Autodesk Inventor part; units mm, degrees
ref_plane "YZ Plane" through (0, 0, 0) normal (1, 0, 0) x (0, 1, 0)
ref_plane "XZ Plane" through (0, 0, 0) normal (0, 1, 0) x (-1, 0, 0)
ref_plane "XY Plane" through (0, 0, 0) normal (0, 0, 1) x (1, 0, 0)
sketch "Sketch1" plane through (0, 0, 0) normal (0, 1, 0) x (-1, 0, 0)
  line L0 (0, 0) -> (6, 0)
  line L1 (6, 0) -> (6, -6)
  line L2 (6, -6) -> (0, -6)
  line L3 (0, -6) -> (0, 0)
  dimension "d0" = 6
extrude "Extrusion1" add sketch "Sketch1" along normal blind 47
sketch "Sketch2" plane through (0, 47, 0) normal (0, 1, 0) x (1, 0, 0)
  line L0 (0, 6) -> (-6, 6)
  line L1 (0, 0) -> (0, 6)
  point P0 (-3, 3)
  point P1 (-3, 6)
  point P2 (0, 3)
  point P3 (-3, 6)
hole "Hole1" at (-3, 47, -3) direction (0, -1, 0) diameter 2.459 depth 10 tip angle 118
sketch "Sketch3" plane through (-6, 47, 0) normal (0, 0, 1) x (1, 0, 0)
  line L0 (0, -47) -> (0, 0)
  line L1 (6, -47) -> (6, 0)
  line L2 (0, 0) -> (6, 0)
  point P0 (3, -47)
  point P1 (3, -15.6667)
  point P2 (0, -94)
  point P3 (6, -94)
  dimension "d17" = 6
  dimension "d18" = 3
  dimension "d19" = 15.6667
  dimension "d20" = 31.3333
  dimension "d21" = 47
hole "Hole2" at (-3, 31.3333, 0) direction (0, 0, -1) diameter 2.459 depth 3 tip angle 118
sketch "Sketch5" plane through (-6, 0, -6) normal (-1, 0, 0) x (0, 0, 1)
  line L0 (0, 0) -> (6, 0)
  point P0 (3, 25)
  point P1 (3, 0)
  dimension "d29" = 25
hole "Hole3" at (-6, 25, -3) direction (1, 0, 0) diameter 2.459 depth 3 tip angle 118
mirror "Mirror2" about plane through (-3, 0, -3) normal (0, -1, 0) of "Extrusion1", "Hole1", "Hole2", "Hole3"
properties part number "VerticalStrut"
CAD build for the part. Positions are in the model's coordinates, mm. A direction names the side the tool comes from. Round coordinates to 2 decimals unless told otherwise and drop trailing zeros. Write each loop counter-clockwise with the first axis right and the second up, starting at its lowest first coordinate (ties: lowest second). Pieces come first, ordered by that corner, then holes. Notation, with made-up numbers: M 5.25,20.25 L 24.25,20.25 A21 ccw 24.25,43.25 Z; hole C 29.25,10.5 d8. An arc over 180 degrees is marked long. Put each result on its own line as item: value. Start each with the question number.
1) Drill centre lines: probe 1 along Y at (x, z) = (-4.9, -3.1); probe 2 along X at (y, z) = (-43, -3); probe 3 along Y at (x, z) = (-5.55, -3.6). Where is each one in solid material? Low to high. Write a range as [from, to].
2) 3-axis set-ups, long thin cutter, end or side, ignore diameter. For faces 1 (the cylindrical face through (-4.48, 26.2, -3.27)), 2 (the cylindrical face through (-4.22, 41.93, -3.16)), 3 (the cylindrical face through (-3.05, 32.56, -1.52)): which of +Z, -Z, +X, -X, +Y, -Y reach the whole face in a straight line?
3) Pull direction Z, two halves, no side cores. Call faces 4 (the conical face through (-3.01, -31.55, -3.61)), 5 (the flat face through (-1.6, 47, -3)), 6 (the flat face through (-3, 1, -6)), 7 (the conical face through (-2.39, -24.82, -2.89)): pulls with the +Z half, pulls with the -Z half, needs draft (parallel to the pull), parting line crosses it, or undercut.
4) Saw through at B-B, the plane x = -5.2. Write the cut outline in (y, z), and give its area (3 significant figures).
5) Saw through at A-A, the plane y = 38. Write the cut outline in (x, z).
6) Pin check, flat tips, straight feed: pin 1 Ø3 at (x, z) = (-3, -3) entering from -Y; pin 2 Ø1.5 at (x, y) = (-3, -31.33) entering from +Z; pin 3 Ø2 at (x, z) = (-3, -3) entering from +Y; pin 4 Ø1.5 at (y, z) = (25, -3) entering from -X. Stop position of each tip, or through.
Resolved:
1. probe 1: [-47, -26.23], [-23.77, 23.77], [26.23, 47]
1. probe 2: [-6, -4.23], [-1.77, 0]
1. probe 3: [-47, -26.07], [-23.93, 23.93], [26.07, 47]
2. face 1: -X
2. face 2: +Y
2. face 3: +Z
3. face 4: pulls with the +Z half
3. face 5: needs draft
3. face 6: pulls with the -Z half
3. face 7: undercut
4. outline: M -47,-6 L 47,-6 L 47,0 L -47,0 Z; hole C -25,-3 d2.46; hole C 25,-3 d2.46
4. area: 555 mm²
5. outline: M -6,-6 L 0,-6 L 0,0 L -6,0 Z; hole C -3,-3 d2.46
6. pin 1: y = -47
6. pin 2: z = -3.29
6. pin 3: y = 36.86
6. pin 4: x = -2.71
